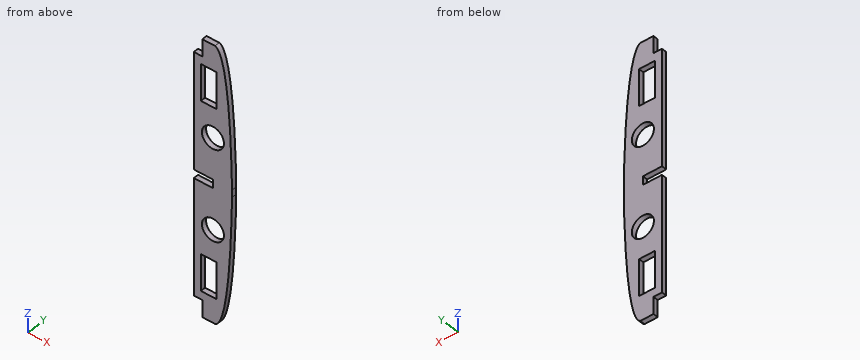
from build123d import *

# Parameters (mm, degrees)
F0_W     = 18.579781
F0_H     = 43.004439
F0_R     = 13.03372
F0_H_2   = 43.004438
F1_DEPTH = 6


with BuildPart() as f1:
    # F0 (on Front) → F1 (new body)
    with BuildSketch(Plane.XZ):
        with BuildLine():
            Line((469.384881, 55.983145), (469.384881, 60.218248))
            Line((469.384881, 60.218248), (446.884881, 60.218248))
            Line((446.884881, 60.218248), (446.884881, 55.218248))
            Line((446.884881, 55.218248), (424.384881, 55.218248))
            Line((424.384881, 55.218248), (424.384881, -81.781752))
            Line((424.384881, -81.781752), (434.384881, -81.781752))
            Line((434.384881, -81.781752), (434.384881, -101.781752))
            Line((434.384881, -101.781752), (449.384881, -101.781752))
            add(Edge.make_bspline(
                [(449.384881, -101.781752), (466.863722, -97.534394), (469.173006, 29.991541), (469.384881, 55.983145)],
                knots=[0, 0, 0, 0, 142.653474, 142.653474, 142.653474, 142.653474], degree=3))
        make_face()
        with Locations((441.996842, -50.5303)):
            Rectangle(F0_W, F0_H, mode=Mode.SUBTRACT)
        with Locations((446.911335, 6.56864)):
            Circle(F0_R, mode=Mode.SUBTRACT)
        with BuildLine():
            add(Edge.make_bspline(
                [(449.384881, 222.218248), (466.863722, 217.97089), (469.173006, 90.444955), (469.384881, 64.453351)],
                knots=[0, 0, 0, 0, 142.653474, 142.653474, 142.653474, 142.653474], degree=3))
            Line((449.384881, 222.218248), (434.384881, 222.218248))
            Line((434.384881, 222.218248), (434.384881, 202.218248))
            Line((434.384881, 202.218248), (424.384881, 202.218248))
            Line((424.384881, 202.218248), (424.384881, 65.218248))
            Line((424.384881, 65.218248), (446.884881, 65.218248))
            Line((446.884881, 65.218248), (446.884881, 60.218248))
            Line((446.884881, 60.218248), (469.384881, 60.218248))
            Line((469.384881, 60.218248), (469.384881, 64.453351))
        make_face()
        with Locations((441.996842, 170.966796)):
            Rectangle(F0_W, F0_H_2, mode=Mode.SUBTRACT)
        with Locations((446.911335, 113.867856)):
            Circle(F0_R, mode=Mode.SUBTRACT)
    extrude(amount=F1_DEPTH)


solid = f1.part
Work out the finished part from the listing and answer in its coordinate system (mm). Give positions to 0.01 mm unless a question says otherwise; leave off trailing zeros. Loops run counter-clockwise (first coordinate to the right, second up) from the corner with the lowest first, then second, coordinate; pieces in that order, holes last. Notation, with made-up numbers: M 24,-24.75 L 50,-24.75 A25 ccw 50,-5.75 Z; hole C 78.25,-0.75 d8. An arc over 180 degrees is marked long. Use CSV: the item, a comma, the result in double quotes.
1) Find section A-A on x = 429.5. Write down the section's boundary in (y, z), plus the area to 3 significant figures.
Answer:
outline,"M -6,-81.78 L 0,-81.78 L 0,55.22 L -6,55.22 Z; M -6,65.22 L 0,65.22 L 0,202.22 L -6,202.22 Z"
area,"1,640 mm^2"
2) Consider L1, parallel to Z at x = 444, y = -3; L2, parallel to Z at x = 448.5, y = -3.5; L3, parallel to Z at x = 455.5, y = -5. Determine where each line is inside the solid, lowest interval first.
Answer:
L1,"-101.78 to -72.03, -29.03 to -6.14, 19.27 to 55.22, 65.22 to 101.16, 126.57 to 149.46, 192.47 to 222.22"
L2,"-101.78 to -72.03, -29.03 to -6.37, 19.51 to 100.93, 126.8 to 149.46, 192.47 to 222.22"
L3,"-94.28 to -3.24, 16.37 to 104.06, 123.67 to 214.71"
3) Given P1, Ø3, axis at x = 429.5, y = -4, coming from the +Z side; P2, Ø6, axis at x = 445.5, z = -42.5, coming from the +Y side; P3, Ø2, axis at x = 431, y = -2.5, coming from the -Z side; P4, Ø3, axis at y = -2.5, z = -91, coming from the -X side, each flat-ended and moving along its own axis, determine where each tip first touches the part or whether it passes through.
Answer:
P1,"z = 202.22"
P2,"through"
P3,"z = -81.78"
P4,"x = 434.38"
4) Find section B-B on x = 443.5. Write down the section's boundary in (y, z).
Answer:
outline,"M -6,-101.78 L 0,-101.78 L 0,-72.03 L -6,-72.03 Z; M -6,-29.03 L 0,-29.03 L 0,-6.01 L -6,-6.01 Z; M -6,19.15 L 0,19.15 L 0,55.22 L -6,55.22 Z; M -6,65.22 L 0,65.22 L 0,101.29 L -6,101.29 Z; M -6,126.45 L 0,126.45 L 0,149.46 L -6,149.46 Z; M -6,192.47 L 0,192.47 L 0,222.22 L -6,222.22 Z"
5) Find section C-C on y = -4. Give the number of separate pieces and of enclosed holes in the cut face, plus the area to 3 significant figures.
Answer:
separate pieces,"1"
enclosed holes,"4"
area,"9,890 mm^2"
